The listing builds one solid part. Answer for the finished solid, in the listing's coordinates (mm). Give positions to 0.01 mm unless a question says otherwise; leave off trailing zeros. Write each loop counter-clockwise with the first axis right and the second up, starting at its lowest first coordinate (ties: lowest second). Pieces come first, ordered by that corner, then holes. Notation, with made-up numbers: (83, 78) - (131, 78) arc R13 cw to (131, 91) - close; hole circle Ø8 at (85.25, -40). An arc over 180 degrees is marked (long way). Answer as CSV lines item,"result". Start each with the question number.
(1) Find section B-B (z = -13.25). Write down the section's boundary in (x, y).
(2) Straight lines are drawn through the part: probe 1 along Z at (x, y) = (0.05, 1.3); probe 2 along X at (y, z) = (0.1, -8.75); probe 3 along X at (y, z) = (-0.25, -2.25). For each, find the intervals that lie inside material, in ascending order.
(3) Each of these flat-tipped pins is pushed along its axis until it touches: pin 1 Ø1.5 at (y, z) = (-1, -4.5) entering from +X; pin 2 Ø1.5 at (x, z) = (-1, 1) entering from +Y (3 decimals); pin 3 Ø1 at (x, y) = (0.5, 1) entering from -Z. Where does it stop, or does it pass through?
(4) Find section A-A (z = 3.25). Write down the section's boundary in (x, y).
(5) For a pull along Z with two mould halves and no side action, classify faces 1 (the face through (-0.19, -0.15, 4.47)), 2 (the face through (0, 0, -16.4)), 3 (the face through (0.86, 0.27, 3.1)) as pulls with the +Z half, pulls with the -Z half, needs draft (parallel to the pull), parting line crosses it, or undercut.
from build123d import *

# Parameters (mm, degrees)
SKETCH1_R                = 0.9
BOSS_EXTRUDE3_DEPTH      = 2.4
BOSS_EXTRUDE4_DEPTH      = 4.7124
BOSS_EXTRUDE4_DEPTH_BACK = 7
SKETCH1_4_R              = 0.9
SKETCH2_R                = 0.5
BOSS_EXTRUDE5_DEPTH      = 9.4
CHAMFER1_SIZE            = 0.9


with BuildPart() as part:
    # Sketch1 → Boss-Extrude3 (new body)
    with BuildSketch(Plane.XY):
        with BuildLine():
            Line((-0.14853508, 1.15297163), (-0.168494904, 1.525812496))
            ThreePointArc((-0.168494904, 1.525812496), (-0.125037571, 1.668563296), (0, 1.75))
            ThreePointArc((0, 1.75), (0.125037571, 1.668563296), (0.168494904, 1.525812496))
            Line((0.168494904, 1.525812496), (0.135913846, 1.154527469))
            ThreePointArc((0.135913846, 1.154527469), (0.294730912, 1.124517647), (0.447850662, 1.072770262))
            Line((0.447850662, 1.072770262), (0.616985381, 1.405639835))
            ThreePointArc((0.616985381, 1.405639835), (0.725995936, 1.507536988), (0.875, 1.515544457))
            ThreePointArc((0.875, 1.515544457), (0.942567361, 1.382499417), (0.908827115, 1.237144931))
            Line((0.908827115, 1.237144931), (0.694968578, 0.931893194))
            ThreePointArc((0.694968578, 0.931893194), (0.817503281, 0.826495394), (0.924235181, 0.705120968))
            Line((0.924235181, 0.705120968), (1.237144931, 0.908827115))
            ThreePointArc((1.237144931, 0.908827115), (1.382499417, 0.942567361), (1.515544457, 0.875))
            ThreePointArc((1.515544457, 0.875), (1.507536988, 0.725995936), (1.405639835, 0.616985381))
            Line((1.405639835, 0.616985381), (1.067807041, 0.459558891))
            ThreePointArc((1.067807041, 0.459558891), (1.121226306, 0.307014366), (1.15297163, 0.14853508))
            Line((1.15297163, 0.14853508), (1.525812496, 0.168494904))
            ThreePointArc((1.525812496, 0.168494904), (1.668563296, 0.125037571), (1.75, 0))
            ThreePointArc((1.75, 0), (1.668563296, -0.125037571), (1.525812496, -0.168494904))
            Line((1.525812496, -0.168494904), (1.154527469, -0.135913846))
            ThreePointArc((1.154527469, -0.135913846), (1.124517647, -0.294730912), (1.072770262, -0.447850662))
            Line((1.072770262, -0.447850662), (1.405639835, -0.616985381))
            ThreePointArc((1.405639835, -0.616985381), (1.507536988, -0.725995936), (1.515544457, -0.875))
            ThreePointArc((1.515544457, -0.875), (1.382499417, -0.942567361), (1.237144931, -0.908827115))
            Line((1.237144931, -0.908827115), (0.931893194, -0.694968578))
            ThreePointArc((0.931893194, -0.694968578), (0.826495394, -0.817503281), (0.705120968, -0.924235181))
            Line((0.705120968, -0.924235181), (0.908827115, -1.237144931))
            ThreePointArc((0.908827115, -1.237144931), (0.942567361, -1.382499417), (0.875, -1.515544457))
            ThreePointArc((0.875, -1.515544457), (0.725995936, -1.507536988), (0.616985381, -1.405639835))
            Line((0.616985381, -1.405639835), (0.459558891, -1.067807041))
            ThreePointArc((0.459558891, -1.067807041), (0.307014366, -1.121226306), (0.14853508, -1.15297163))
            Line((0.14853508, -1.15297163), (0.168494904, -1.525812496))
            ThreePointArc((0.168494904, -1.525812496), (0.125037571, -1.668563296), (0, -1.75))
            ThreePointArc((0, -1.75), (-0.125037571, -1.668563296), (-0.168494904, -1.525812496))
            Line((-0.168494904, -1.525812496), (-0.135913846, -1.154527469))
            ThreePointArc((-0.135913846, -1.154527469), (-0.294730912, -1.124517647), (-0.447850662, -1.072770262))
            Line((-0.447850662, -1.072770262), (-0.616985381, -1.405639835))
            ThreePointArc((-0.616985381, -1.405639835), (-0.725995936, -1.507536988), (-0.875, -1.515544457))
            ThreePointArc((-0.875, -1.515544457), (-0.942567361, -1.382499417), (-0.908827115, -1.237144931))
            Line((-0.908827115, -1.237144931), (-0.694968578, -0.931893194))
            ThreePointArc((-0.694968578, -0.931893194), (-0.817503281, -0.826495394), (-0.924235181, -0.705120968))
            Line((-0.924235181, -0.705120968), (-1.237144931, -0.908827115))
            ThreePointArc((-1.237144931, -0.908827115), (-1.382499417, -0.942567361), (-1.515544457, -0.875))
            ThreePointArc((-1.515544457, -0.875), (-1.507536988, -0.725995936), (-1.405639835, -0.616985381))
            Line((-1.405639835, -0.616985381), (-1.067807041, -0.459558891))
            ThreePointArc((-1.067807041, -0.459558891), (-1.121226306, -0.307014366), (-1.15297163, -0.14853508))
            Line((-1.15297163, -0.14853508), (-1.525812496, -0.168494904))
            ThreePointArc((-1.525812496, -0.168494904), (-1.668563296, -0.125037571), (-1.75, 0))
            ThreePointArc((-1.75, 0), (-1.668563296, 0.125037571), (-1.525812496, 0.168494904))
            Line((-1.525812496, 0.168494904), (-1.154527469, 0.135913846))
            ThreePointArc((-1.154527469, 0.135913846), (-1.124517647, 0.294730912), (-1.072770262, 0.447850662))
            Line((-1.072770262, 0.447850662), (-1.405639835, 0.616985381))
            ThreePointArc((-1.405639835, 0.616985381), (-1.507536988, 0.725995936), (-1.515544457, 0.875))
            ThreePointArc((-1.515544457, 0.875), (-1.382499417, 0.942567361), (-1.237144931, 0.908827115))
            Line((-1.237144931, 0.908827115), (-0.931893194, 0.694968578))
            ThreePointArc((-0.931893194, 0.694968578), (-0.826495394, 0.817503281), (-0.705120968, 0.924235181))
            Line((-0.705120968, 0.924235181), (-0.908827115, 1.237144931))
            ThreePointArc((-0.908827115, 1.237144931), (-0.942567361, 1.382499417), (-0.875, 1.515544457))
            ThreePointArc((-0.875, 1.515544457), (-0.725995936, 1.507536988), (-0.616985381, 1.405639835))
            Line((-0.616985381, 1.405639835), (-0.459558891, 1.067807041))
            ThreePointArc((-0.459558891, 1.067807041), (-0.307014366, 1.121226306), (-0.14853508, 1.15297163))
        make_face()
        Circle(SKETCH1_R, mode=Mode.SUBTRACT)
    extrude(amount=BOSS_EXTRUDE3_DEPTH)

    # Sketch1_4 → Boss-Extrude4 (add, two sides: drawn at the far end of the back side and taken through both)
    with BuildSketch(Plane.XY.offset(-BOSS_EXTRUDE4_DEPTH_BACK)):
        Circle(SKETCH1_4_R)
    extrude(amount=BOSS_EXTRUDE4_DEPTH + BOSS_EXTRUDE4_DEPTH_BACK)

    # Sketch2 → Boss-Extrude5 (add)
    with BuildSketch(Plane(origin=(0, 0, -7), x_dir=(-1, 0, 0), z_dir=(0, 0, -1))):
        with Locations(Location((0, 0, 0), (0, 0, 180))):
            Circle(SKETCH2_R)
    extrude(amount=BOSS_EXTRUDE5_DEPTH)

    # Chamfer1
    chamfer1_edges = [part.edges().sort_by_distance(p)[0] for p in [
        (-0.9, 0, 4.7124),
    ]]
    chamfer(chamfer1_edges, length=CHAMFER1_SIZE)


solid = part.part
Result set:
1,outline,"circle Ø1 at (0, 0)"
2,probe 1,"0 to 2.4"
2,probe 2,"-0.49 to 0.49"
2,probe 3,"-0.86 to 0.86"
3,pin 1,"x = 0.86"
3,pin 2,"y = 1.525"
3,pin 3,"z = -7"
4,outline,"circle Ø1.8 at (0, 0)"
5,face 1,"pulls with the +Z half"
5,face 2,"pulls with the -Z half"
5,face 3,"needs draft"
